Verification items for this drawing (mm, ordinates from the low corner). Round coordinates to 2 decimals unless told otherwise and drop trailing zeros. Write each loop counter-clockwise with the first axis right and the second up, starting at its lowest first coordinate (ties: lowest second). Pieces come first, ordered by that corner, then holes. Notation, with made-up numbers: M 89.5,-22 L 101.5,-22 A31 ccw 101.5,17 Z; hole C -19.5,-31 d9. An arc over 180 degrees is marked long. One line per question, with ' | ' between items. Start each with the question number.
Q1. Cross-section at C-C (y = 6). Record the boundary of the cut face in (x, z) (1 decimal), then the cut area to 3 significant figures.
Q2. Release check for a two-part mould opening along Z. For the marked faces 1, 2 and 3 record: released by +Z, released by -Z, zero draft, split by the parting line, or undercut.
Q3. Cross-section at A-A (z = 14.25). Record the boundary of the cut face in (x, y) (1 decimal).
Q4. Cross-section at D-D (x = 19.25). Record the boundary of the cut face in (y, z).
Q5. Cross-section at B-B (x = 6). Record the boundary of the cut face in (y, z).
Q6. Gauge pin test, flat ends, axial feed: pin 1 (2 mm diameter, centred on x = 15, y = 5, fed in from +Z); pin 2 (2 mm diameter, centred on y = 3.5, z = 13.5, fed in from -X); pin 3 (3 mm diameter, centred on x = 13.5, y = 2.5, fed in from -Z). Record the tip position at first contact, or that the pin passes through.
Q7. Thickness scan on line 1 along X through (y, z) = (5.5, 11.25) (1 decimal); line 2 along Z through (x, y) = (6.25, 6) (1 decimal); line 3 along Z through (x, y) = (11, 6.75) (1 decimal). Record the ranges inside material, lowest first. Write a range as from..to.
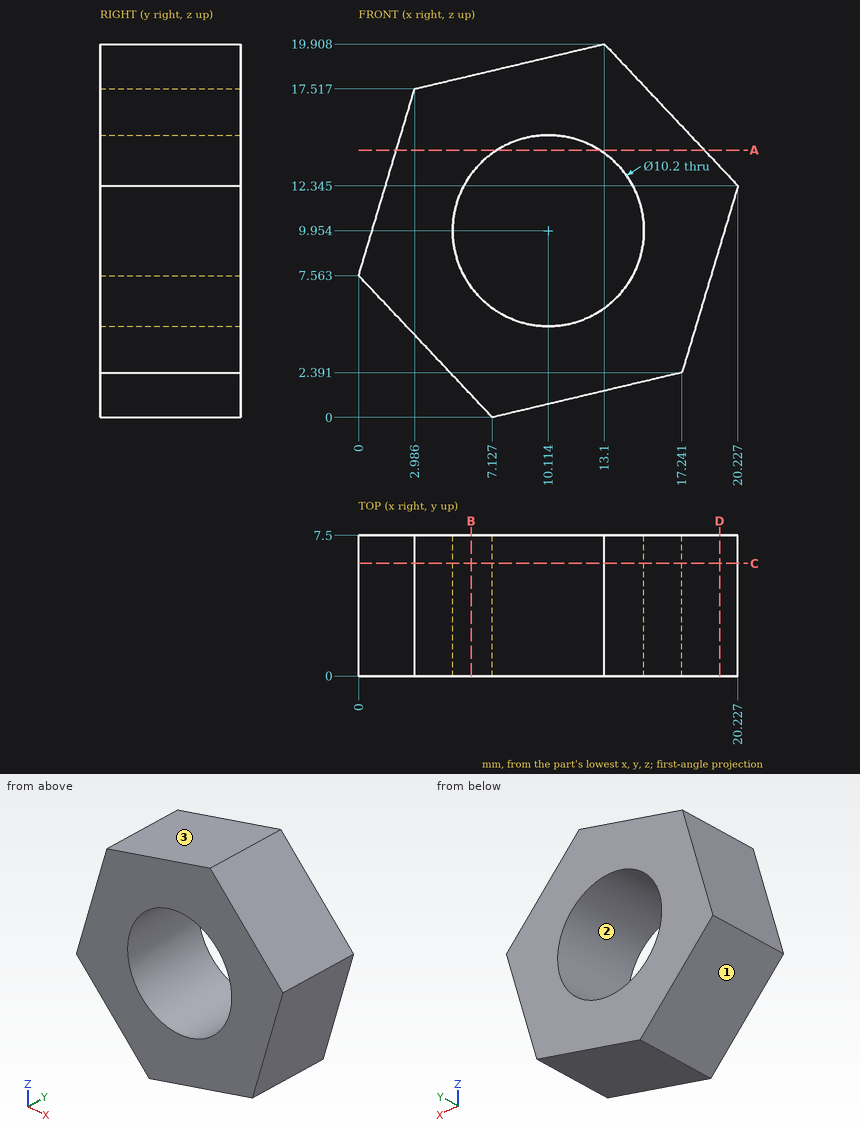
Determined:
1) outline: M 0,7.6 L 7.1,0 L 17.2,2.4 L 20.2,12.3 L 13.1,19.9 L 3,17.5 Z; hole C 10.1,10 d10.2 | area: 199 mm²
2) face 1: released by -Z | face 2: undercut | face 3: released by +Z
3) outline: M 2,0 L 7.4,0 L 7.4,7.5 L 2,7.5 Z; M 12.9,0 L 18.4,0 L 18.4,7.5 L 12.9,7.5 Z
4) outline: M 0,9.09 L 7.5,9.09 L 7.5,13.38 L 0,13.38 Z
5) outline: M 0,1.2 L 7.5,1.2 L 7.5,6.94 L 0,6.94 Z; M 0,12.97 L 7.5,12.97 L 7.5,18.23 L 0,18.23 Z
6) pin 1: stops at z = 18.95 | pin 2: stops at x = 1.48 | pin 3: stops at z = 1.15
7) line 1: x = 1.1..5.2, 15..19.9 | line 2: z = 0.9..6.6, 13.3..18.3 | line 3: z = 0.9..4.9, 15..19.4
